Verification items for the finished model (mm, model axes). Face numbers are marked on the shaded views. Give positions to 0.01 mm unless a question says otherwise; leave off trailing zeros. Write each loop counter-clockwise with the first axis right and the second up, starting at its lowest first coordinate (ties: lowest second). Pieces come first, ordered by that corner, then holes. Notation, with made-up numbers: M 48.25,-27 L 94.25,-27 A4 ccw 94.25,-20 Z; hole C 73,59.5 d4. An arc over 180 degrees is marked long. Answer as a JSON object with one key per item and string values.
```python
from build123d import *

# Parameters (mm, degrees)
SKETCH1_R           = 6
SKETCH1_R_2         = 4
BOSS_EXTRUDE1_DEPTH = 10
SKETCH2_R           = 1
CUT_EXTRUDE1_DEPTH  = 10


with BuildPart() as part:
    # Sketch1 → Boss-Extrude1 (new, symmetric)
    with BuildSketch(Plane.XY):
        Circle(SKETCH1_R)
        Circle(SKETCH1_R_2, mode=Mode.SUBTRACT)
    extrude(amount=BOSS_EXTRUDE1_DEPTH, both=True)

    # Sketch2 → Cut-Extrude1 (cut, symmetric)
    with BuildSketch(Plane(origin=(0, 0, 0), x_dir=(0, 0, -1), z_dir=(1, 0, 0))):
        with Locations((-6, 0)):
            Circle(SKETCH2_R)
    cut_extrude1 = extrude(amount=CUT_EXTRUDE1_DEPTH, both=True, mode=Mode.SUBTRACT)

    # Mirror1: Cut-Extrude1 across plane
    add(cut_extrude1.mirror(Plane.XY), mode=Mode.SUBTRACT)


solid = part.part
```
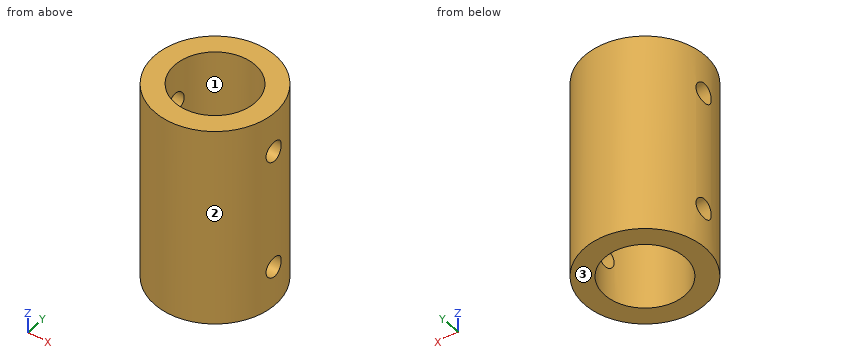
1) Thickness scan on L1, parallel to Z at x = 5.55, y = 0; L2, parallel to X at y = 0, z = -1; L3, parallel to X at y = 2, z = 0.75. Record the ranges inside material, lowest first.
Completed:
{"L1": "z = -10 to -7, -5 to 5, 7 to 10", "L2": "x = -6 to -4, 4 to 6", "L3": "x = -5.66 to -3.46, 3.46 to 5.66"}
2) Section check A-A on y = 0. Record the boundary of the cut face in (x, z).
Completed:
{"outline": "M -6,-10 L -4,-10 L -4,-7 L -6,-7 Z; M -6,-5 L -4,-5 L -4,5 L -6,5 Z; M -6,7 L -4,7 L -4,10 L -6,10 Z; M 4,-10 L 6,-10 L 6,-7 L 4,-7 Z; M 4,-5 L 6,-5 L 6,5 L 4,5 Z; M 4,7 L 6,7 L 6,10 L 4,10 Z"}
3) Section check D-D on x = -5. Record the boundary of the cut face in (y, z).
Completed:
{"outline": "M -3.32,-10 L 3.32,-10 L 3.32,10 L -3.32,10 Z; hole C 0,-6 d2; hole C 0,6 d2"}
4) Section check C-C on y = 2. Record the boundary of the cut face in (x, z).
Completed:
{"outline": "M -5.66,-10 L -3.46,-10 L -3.46,10 L -5.66,10 Z; M 3.46,-10 L 5.66,-10 L 5.66,10 L 3.46,10 Z"}
5) Release check for a two-part mould opening along X. For the marked faces 1, 2 and 3 record: pulls with the +X half, pulls with the -X half, needs draft (parallel to the pull), parting line crosses it, or undercut.
Completed:
{"face 1": "undercut", "face 2": "parting line crosses it", "face 3": "needs draft"}
6) Section check B-B on x = 0. Record the boundary of the cut face in (y, z), and give its area (3 significant figures).
Completed:
{"outline": "M -6,-10 L -4,-10 L -4,10 L -6,10 Z; M 4,-10 L 6,-10 L 6,10 L 4,10 Z", "area": "80.0 mm2"}
7) Go/stop test with flat-tipped pins: pin 1 (1 mm diameter, centred on x = 4, z = 0.5, fed in from +Y); pin 2 (1.6 mm diameter, centred on y = 0, z = 6, fed in from +X). Record where each tip stops, or that it passes through.
Completed:
{"pin 1": "stops at y = 4.87", "pin 2": "passes through"}
